from build123d import *

# Parameters (mm, degrees)
F0_W     = 136
F0_H     = 50
F1_DEPTH = 25
F2_W     = 128
F2_H     = 10
F3_DEPTH = 25.001
F4_R     = 2


with BuildPart() as f1:
    # F0 (on Front) → F1 (new body)
    with BuildSketch(Plane.XZ):
        Rectangle(F0_W, F0_H)
    extrude(amount=F1_DEPTH)

    # F2 (on face) → F3 (cut, through all)
    with BuildSketch(Plane.XZ.offset(25)):
        with Locations((0, 20)):
            Rectangle(F2_W, F2_H)
    extrude(amount=-F3_DEPTH, mode=Mode.SUBTRACT)

    # F4
    f4_edges = [f1.edges().sort_by_distance(p)[0] for p in [
        (-64, -12.5, 25),
        (64, -12.5, 25),
    ]]
    fillet(f4_edges, radius=F4_R)


solid = f1.part
The listing builds one solid part. Answer for the finished solid, in the listing's coordinates (mm). A direction names the side the tool comes from. Round coordinates to 2 decimals unless told otherwise and drop trailing zeros. Write each loop counter-clockwise with the first axis right and the second up, starting at its lowest first coordinate (ties: lowest second). Pieces come first, ordered by that corner, then holes. Notation, with made-up numbers: (-8.75, 34.25) - (35.25, 34.25) arc R22 ccw to (35.25, 53.25) - close; hole circle Ø1 at (43.5, 7). An arc over 180 degrees is marked (long way). Use one line per item in the form item = value. Start each with the question number.
Item 1: A cutting plane is placed at C-C (x = -43). Write down the section's boundary in (y, z).
Item 2: Find the intervals of material crossed by line 1 (X direction, y = -2.75, z = 18); line 2 (Z direction, x = -14.5, y = -17), in increasing order. Write a range as [from, to].
Item 3: A flat-ended cylindrical pin translates along its axis: pin 1 Ø7.5 at (x, y) = (5.5, -14) entering from +Z. Find the tip coordinate at first contact, or state that the pin passes through.
Item 4: A cutting plane is placed at A-A (z = 17). Write down the section's boundary in (x, y), plus the area to 3 significant figures.
Item 5: Determine the mould class of faces 1 (the flat face through (64, -13, 19)), 2 (the flat face through (68, -12, 0)), 3 (the flat face through (-1, -25, -5)), 4 (the flat face through (-64, -13, 19)) for opening direction X: +X half, -X half, draft (parallel to the pull), parting line (faces both ways), or undercut.
Item 6: A cutting plane is placed at B-B (y = -11.5). Write down the section's boundary in (x, z).
Item 7: A tool of negligible diameter and unlimited length cuts with its end or side. For faces 5 (the flat face through (-68, -12, 0)), 6 (the flat face through (-1, -13, 15)), from which of +Z, -Z, +X, -X, +Y, -Y can it reach the whole face along a straight path? Write none if from no direction.
The answers:
q1.outline = (-25, -25) - (0, -25) - (0, 15) - (-25, 15) - close
q2.line_1 = [-68, -64], [64, 68]
q2.line_2 = [-25, 15]
q3.pin_1 = 15
q4.outline = (-68, -25) - (-64, -25) - (-64, 0) - (-68, 0) - close; (64, -25) - (68, -25) - (68, 0) - (64, 0) - close
q4.area = 200 mm^2
q5.face_1 = undercut
q5.face_2 = +X half
q5.face_3 = draft
q5.face_4 = undercut
q6.outline = (-68, -25) - (68, -25) - (68, 25) - (66, 25) arc R2 ccw to (64, 23) - (64, 15) - (-64, 15) - (-64, 23) arc R2 ccw to (-66, 25) - (-68, 25) - close
q7.face_5 = +Z, -Z, -X, +Y, -Y
q7.face_6 = +Z, +Y, -Y
